Source: CAD feature listing. Evaluate the final solid. Frame: model axes, mm. Give positions to 0.01 mm unless a question says otherwise; leave off trailing zeros. Order: outer loops, then holes, each group sorted by start corner. A loop starts at its lowest first (then second) coordinate and runs counter-clockwise, first axis right, second up.
from build123d import *

# Parameters (mm, degrees)
SKETCH1_R           = 12.5
BOSS_EXTRUDE1_DEPTH = 10


with BuildPart() as part:
    # Sketch1 → Boss-Extrude1 (new body)
    with BuildSketch(Plane.XY):
        with BuildLine():
            Line((0, 35), (700, 35))
            ThreePointArc((700, 35), (735, 0), (700, -35))
            Line((700, -35), (0, -35))
            ThreePointArc((0, -35), (-35, 0), (0, 35))
        make_face()
        Circle(SKETCH1_R, mode=Mode.SUBTRACT)
        with Locations((50, 0)):
            Circle(SKETCH1_R, mode=Mode.SUBTRACT)
        with Locations((100, 0)):
            Circle(SKETCH1_R, mode=Mode.SUBTRACT)
        with Locations((150, 0)):
            Circle(SKETCH1_R, mode=Mode.SUBTRACT)
        with Locations((200, 0)):
            Circle(SKETCH1_R, mode=Mode.SUBTRACT)
        with Locations((250, 0)):
            Circle(SKETCH1_R, mode=Mode.SUBTRACT)
        with Locations((300, 0)):
            Circle(SKETCH1_R, mode=Mode.SUBTRACT)
        with Locations((350, 0)):
            Circle(SKETCH1_R, mode=Mode.SUBTRACT)
        with Locations((400, 0)):
            Circle(SKETCH1_R, mode=Mode.SUBTRACT)
        with Locations((450, 0)):
            Circle(SKETCH1_R, mode=Mode.SUBTRACT)
        with Locations((500, 0)):
            Circle(SKETCH1_R, mode=Mode.SUBTRACT)
        with Locations((550, 0)):
            Circle(SKETCH1_R, mode=Mode.SUBTRACT)
        with Locations((600, 0)):
            Circle(SKETCH1_R, mode=Mode.SUBTRACT)
        with Locations((650, 0)):
            Circle(SKETCH1_R, mode=Mode.SUBTRACT)
        with Locations((700, 0)):
            Circle(SKETCH1_R, mode=Mode.SUBTRACT)
    extrude(amount=BOSS_EXTRUDE1_DEPTH)


solid = part.part
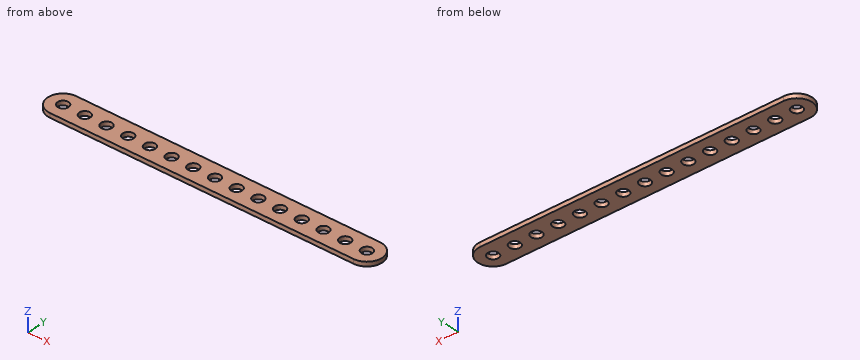
(1) Section D-D, the plane y = 27. Return loops of the section in (x, z).
(2) Pin query (flat end, axial travel): pin 1 Ø22.5 at (x, y) = (650, 0) entering from -Z; pin 2 Ø2 at (y, z) = (-27.5, 5) entering from +X; pin 3 Ø5 at (y, z) = (23, 8.5) entering from +X. Return the tip coordinate at first contact, or that it passes through.
(3) Section C-C, the plane x = 601. Return loops of the section in (y, z), plus the area to 3 significant figures.
(4) Section A-A, the plane x = 150. Return loops of the section in (y, z).
(5) Line query: line 1 along Y through (x, z) = (700, 6); line 2 along Y through (x, z) = (595.5, 8); line 3 along X through (y, z) = (27, 8.75). Output: solid intervals per line, ascending.
(6) Section B-B, the plane z = 6. Count the separate pieces of the cut face and the enclosed holes in it, plus the area to 3 significant figures.
Checks:
1. outline: (-22.27, 0) - (722.27, 0) - (722.27, 10) - (-22.27, 10) - close
2. pin 1: passes through
2. pin 2: stops at x = 722.86
2. pin 3: stops at x = 728.37
3. outline: (-35, 0) - (-12.46, 0) - (-12.46, 10) - (-35, 10) - close; (12.46, 0) - (35, 0) - (35, 10) - (12.46, 10) - close
3. area: 451 mm2
4. outline: (-35, 0) - (-12.5, 0) - (-12.5, 10) - (-35, 10) - close; (12.5, 0) - (35, 0) - (35, 10) - (12.5, 10) - close
5. line 1: y = -35 to -12.5, 12.5 to 35
5. line 2: y = -35 to -11.66, 11.66 to 35
5. line 3: x = -22.27 to 722.27
6. separate pieces: 1
6. enclosed holes: 15
6. area: 45,500 mm2
